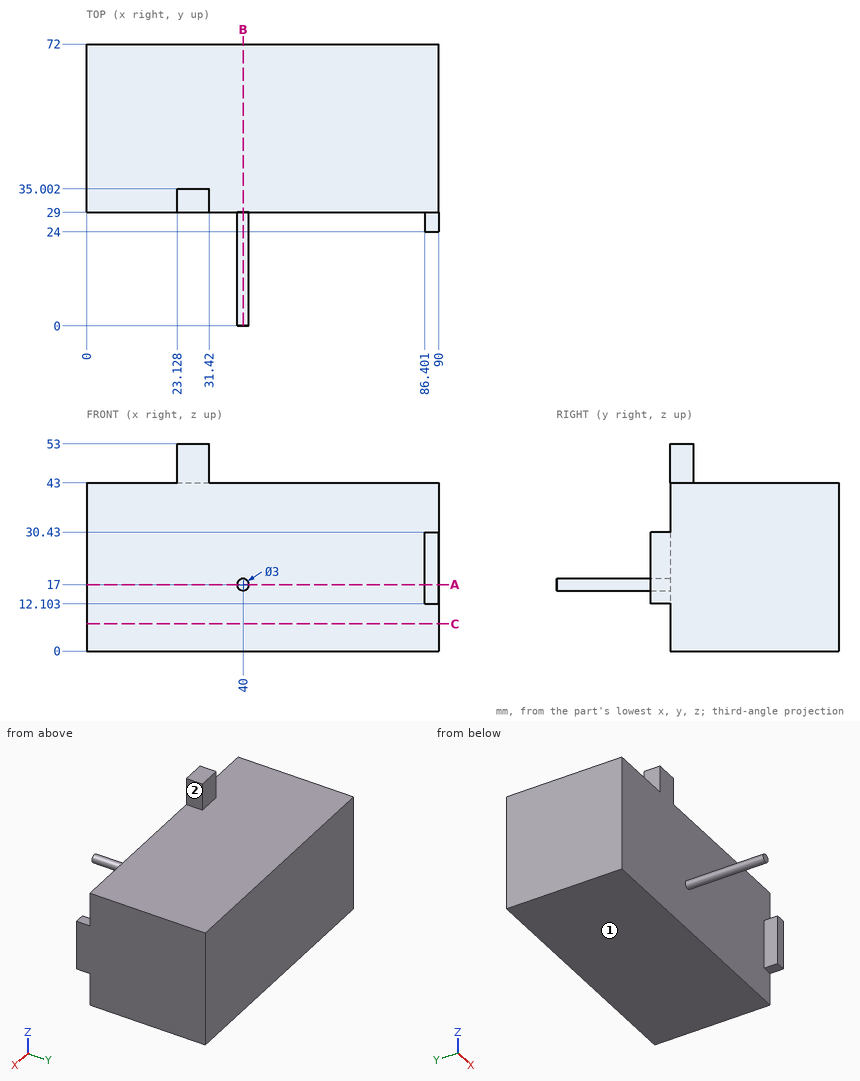
Could you check a few things on this drawing? It's one solid part, dimensions in mm from its lowest x, y, z. A direction names the side the tool comes from. Coordinates: 2 decimals unless noted, no trailing zeros. Order: outer loops, then holes, each group sorted by start corner. A loop starts at its lowest first (then second) coordinate and runs counter-clockwise, first axis right, second up. Notation, with made-up numbers: (74.25, 1.25) -> (127.25, 1.25) arc R32 cw to (127.25, 36.25) -> close; hole circle Ø2 at (73.5, 63). An arc over 180 degrees is marked (long way). One line per item, written item: value. Start each with the question number.
1) Which directions (+Z, -Z, +X, -X, +Y, -Y) give clear straight access to the entire face, cutting with the end or side of a thin tool? Please do the marked faces 1 and 2.
2) Imagine slicing it at A-A on z = 17. List the corners of the cut face in (x, y) for me.
3) Imagine slicing it at C-C on z = 7. List the corners of the cut face in (x, y) for me, plus the area to 3 significant figures.
4) I'm going to push flat-ended pins straight in: pin 1 (3 mm diameter, centred on x = 88, z = 22, fed in from -Y); pin 2 (12 mm diameter, centred on x = 70.5, z = 13.5, fed in from -Y); pin 3 (2.5 mm diameter, centred on y = 27, z = 23, fed in from -X). Where does each tip first touch, or does it pass through?
5) Imagine slicing it at B-B on x = 40. List the corners of the cut face in (y, z) for me.
6) If I drill on L1, parallel to Y at x = 5.5, z = 21; L2, parallel to Z at x = 67, y = 45.5; L3, parallel to X at y = 32.5, z = 49, over which ranges is the centre line in solid material (lowest first)? Write a range as [from, to].
Answer list:
1. face 1: -Z, +X, -X, +Y, -Y
1. face 2: +Z, +X, +Y, -Y
2. outline: (0, 29) -> (38.5, 29) -> (38.5, 0) -> (41.5, 0) -> (41.5, 29) -> (86.4, 29) -> (86.4, 24) -> (90, 24) -> (90, 72) -> (0, 72) -> close
3. outline: (0, 29) -> (90, 29) -> (90, 72) -> (0, 72) -> close
3. area: 3,870 mm2
4. pin 1: stops at y = 24
4. pin 2: stops at y = 29
4. pin 3: stops at x = 86.4
5. outline: (0, 15.5) -> (29, 15.5) -> (29, 0) -> (72, 0) -> (72, 43) -> (29, 43) -> (29, 18.5) -> (0, 18.5) -> close
6. L1: y = [29, 72]
6. L2: z = [0, 43]
6. L3: x = [23.13, 31.42]
